Could you check a few things on this drawing? It's one solid part, dimensions in mm from its lowest x, y, z. A direction names the side the tool comes from. Coordinates: 2 decimals unless noted, no trailing zeros. Write each loop counter-clockwise with the first axis right and the second up, starting at its lowest first coordinate (ties: lowest second). Pieces come first, ordered by that corner, then holes. Notation, with made-up numbers: M 14,-22.75 L 66,-22.75 A16 cw 66,4.25 Z; hole C -28.75,-1.5 d10. An arc over 180 degrees is marked long. Use a Markdown table: item, result.
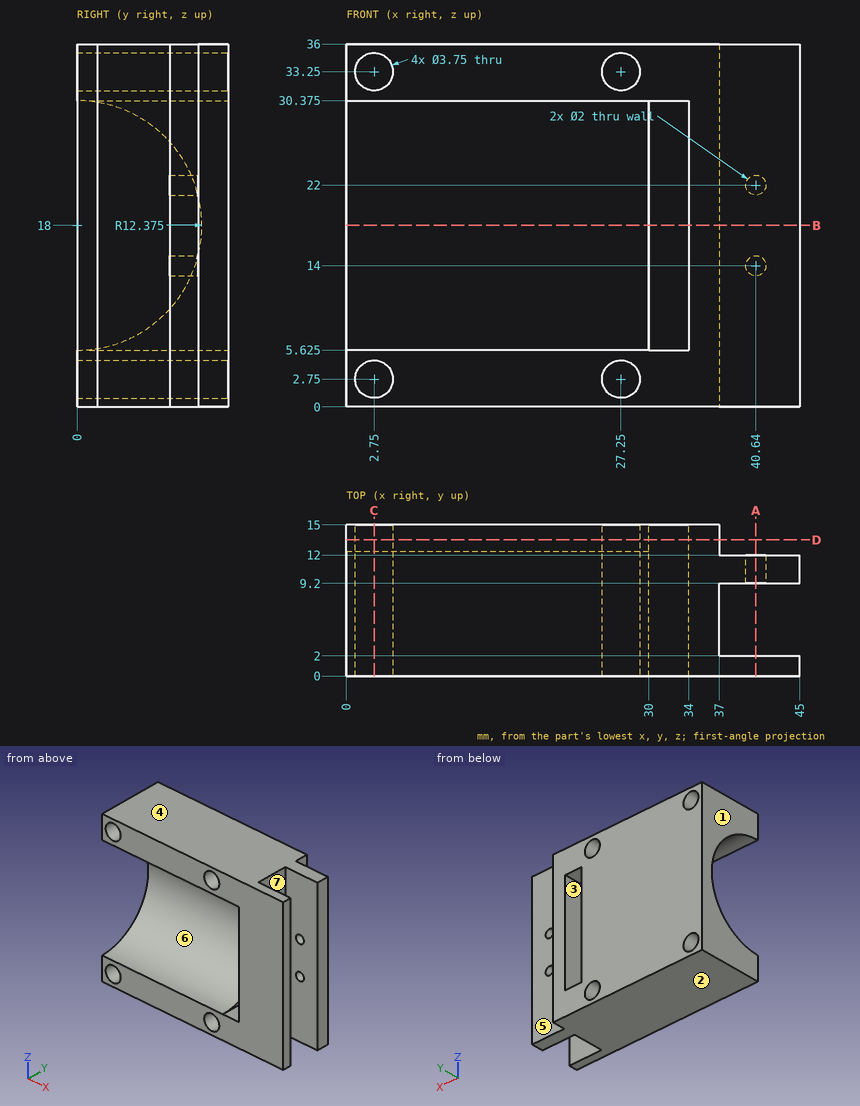
1. I need wall thicknesses on probe 1 along X at (y, z) = (9, 2.75) (3 decimals); probe 2 along Z at (x, y) = (40.64, 10.4); probe 3 along Y at (x, z) = (41.5, 34). Which ranges of each line are inside material? Lowest first, please.
Answers follow:
| item | result |
|---|---|
| probe 1 | x = 0 to 0.875, 4.625 to 25.375, 29.125 to 37 |
| probe 2 | z = 0 to 13, 15 to 21, 23 to 36 |
| probe 3 | y = 0 to 2, 9.2 to 12 |
2. Suppose I cut it at C-C on x = 2.75. Write out the boundary of the cut face in (y, z) (3 decimals), and give its area (3 significant figures).
Answers follow:
| item | result |
|---|---|
| outline | M 0,0 L 15,0 L 15,0.875 L 0,0.875 Z; M 0,4.625 L 15,4.625 L 15,31.375 L 0,31.375 L 0,30.375 A12.375 cw 0,5.625 Z; M 0,35.125 L 15,35.125 L 15,36 L 0,36 Z |
| area | 187 mm2 |
3. Suppose I cut it at A-A on x = 40.64. Write out the boundary of the cut face in (y, z), and give its area (3 significant figures).
Answers follow:
| item | result |
|---|---|
| outline | M 0,0 L 2,0 L 2,36 L 0,36 Z; M 9.2,0 L 12,0 L 12,13 L 9.2,13 Z; M 9.2,15 L 12,15 L 12,21 L 9.2,21 Z; M 9.2,23 L 12,23 L 12,36 L 9.2,36 Z |
| area | 162 mm2 |
4. Which directions (+Z, -Z, +X, -X, +Y, -Y) give clear straight access to the entire face, cutting with the end or side of a thin tool? Please do the marked faces 5, 6 and 7.
Answers follow:
| item | result |
|---|---|
| face 5 | +Z, -Z, +X, +Y |
| face 6 | -X, -Y |
| face 7 | +Z, -Z, +X |
5. Suppose I cut it at D-D on y = 13.5. Write out the boundary of the cut face in (x, z) (3 decimals), and give its area (3 significant figures).
Answers follow:
| item | result |
|---|---|
| outline | M 0,0 L 37,0 L 37,36 L 0,36 Z; hole C 2.75,2.75 d3.75; hole C 2.75,33.25 d3.75; hole C 27.25,2.75 d3.75; hole C 27.25,33.25 d3.75; hole M 30,5.625 L 34,5.625 L 34,30.375 L 30,30.375 Z |
| area | 1,190 mm2 |
6. Will these pins go through, and if not, where does the flat tip stop? pin 1 Ø1.5 at (y, z) = (13, 10.5) entering from +X; pin 2 Ø2.5 at (x, z) = (43, 15) entering from +Y; pin 3 Ø7.5 at (y, z) = (4.5, 23) entering from -X.
Answers follow:
| item | result |
|---|---|
| pin 1 | stops at x = 37 |
| pin 2 | stops at y = 12 |
| pin 3 | stops at x = 34 |
7. We'd pull the mould along Z, two halves only. Please class the marked faces 1, 2, 3 and 4: +Z half, -Z half, draft (parallel to the pull), parting line (faces both ways), or undercut.
Answers follow:
| item | result |
|---|---|
| face 1 | draft |
| face 2 | -Z half |
| face 3 | undercut |
| face 4 | +Z half |
8. Suppose I cut it at B-B on z = 18. Write out the boundary of the cut face in (x, y) (3 decimals).
Answers follow:
| item | result |
|---|---|
| outline | M 0,12.375 L 30,12.375 L 30,15 L 0,15 Z; M 34,0 L 45,0 L 45,2 L 37,2 L 37,9.2 L 45,9.2 L 45,12 L 37,12 L 37,15 L 34,15 Z |
